Geometry: final body of the model. Coordinates: model frame, mm. A direction names the side the tool comes from. Coordinates: 2 decimals unless noted, no trailing zeros. Order: outer loops, then holes, each group sorted by start corner. A loop starts at its lowest first (then second) coordinate and runs counter-clockwise, first axis right, second up. Notation, with made-up numbers: (75, 84.5) - (80, 84.5) arc R24 ccw to (80, 123.5) - close; hole circle Ø6 at (49, -28.5). An arc over 180 degrees is marked (long way). Use one line per item in the form item = value. Start each with the question number.
```python
from build123d import *

# Parameters (mm, degrees)
ESQUISSE1_W        = 12.45
ESQUISSE1_H        = 2.1
BOSS_EXTRU_1_DEPTH = 8.4
ESQUISSE2_W        = 12.45
ESQUISSE2_H        = 30.368041495
BOSS_EXTRU_2_DEPTH = 3
CONG_1_R           = 2


with BuildPart() as part:
    # Esquisse1 → Boss.-Extru.1 (new body)
    with BuildSketch(Plane.XY):
        with Locations((6.225, 1.05)):
            Rectangle(ESQUISSE1_W, ESQUISSE1_H)
    extrude(amount=BOSS_EXTRU_1_DEPTH)

    # Esquisse2 → Boss.-Extru.2 (add)
    with BuildSketch(Plane.XY.offset(8.4)):
        with Locations((6.225, 1.097662534)):
            Rectangle(ESQUISSE2_W, ESQUISSE2_H)
    extrude(amount=BOSS_EXTRU_2_DEPTH)

    # Congé1
    cong_1_edges = [part.edges().sort_by_distance(p)[0] for p in [
        (12.45, -14.086358213, 9.9),
        (12.45, 16.281683282, 9.9),
        (0, 16.281683282, 9.9),
        (0, -14.086358213, 9.9),
    ]]
    fillet(cong_1_edges, radius=CONG_1_R)


solid = part.part
```
(1) Material intervals for L1, parallel to Z at x = 3, y = 12; L2, parallel to Y at x = 1.5, z = 7.5; L3, parallel to Y at x = 11.75, z = 8.5, sorted ascending. Write a range as from..to.
(2) Contact query for flat-ended pins moving along their axis: pin 1 Ø3.5 at (x, y) = (6, 7) entering from -Z; pin 2 Ø2.5 at (x, z) = (5.5, 5.5) entering from +Y; pin 3 Ø6 at (y, z) = (-8, 4) entering from +X; pin 4 Ø2 at (x, z) = (4.5, 4) entering from -Y. Output: stop coordinate, or through.
(3) Cut plane D-D on x = 11. Return the cut outline in (y, z).
(4) Cut plane C-C on z = 8. Return the cut outline in (x, y), plus the area to 3 significant figures.
(5) Cut plane A-A on x = 4. Return the cut outline in (y, z).
(6) Cut plane B-B on y = 3.5. Return the cut outline in (x, z), plus the area to 4 significant figures.
(7) Draft query along X for faces 4 (the cylindrical face through (11.849, -13.516, 9.921)), 5 (the cylindrical face through (0.57, 15.68, 9.92)), 6 (the flat face through (6, -7, 8.4)). Return one class per face: released by +X, released by -X, zero draft, split by the parting line, or undercut.
(8) Set-up query: faces 1 (the flat face through (12.45, 1, 9)), 2 (the flat face through (6, 2.1, 4)), 3 (the flat face through (6, 0, 4)). Return all of +Z, -Z, +X, -X, +Y, -Y with unobstructed straight access to the full face (end or side cutting, diameter ignored); none if empty.
Check sheet entries:
q1.L1 = 8.4..11.4
q1.L2 = 0..2.1
q1.L3 = -13.61..15.8
q2.pin_1 = 8.4
q2.pin_2 = 2.1
q2.pin_3 = through
q2.pin_4 = 0
q3.outline = (-14.01, 8.4) - (0, 8.4) - (0, 0) - (2.1, 0) - (2.1, 8.4) - (16.2, 8.4) - (16.2, 11.4) - (-14.01, 11.4) - close
q4.outline = (0, 0) - (12.45, 0) - (12.45, 2.1) - (0, 2.1) - close
q4.area = 26.1 mm^2
q5.outline = (-14.09, 8.4) - (0, 8.4) - (0, 0) - (2.1, 0) - (2.1, 8.4) - (16.28, 8.4) - (16.28, 11.4) - (-14.09, 11.4) - close
q6.outline = (0, 8.4) - (12.45, 8.4) - (12.45, 11.4) - (0, 11.4) - close
q6.area = 37.35 mm^2
q7.face_4 = released by +X
q7.face_5 = released by -X
q7.face_6 = zero draft
q8.face_1 = +Z, -Z, +X, +Y, -Y
q8.face_2 = -Z, +X, -X, +Y
q8.face_3 = -Z, +X, -X, -Y
